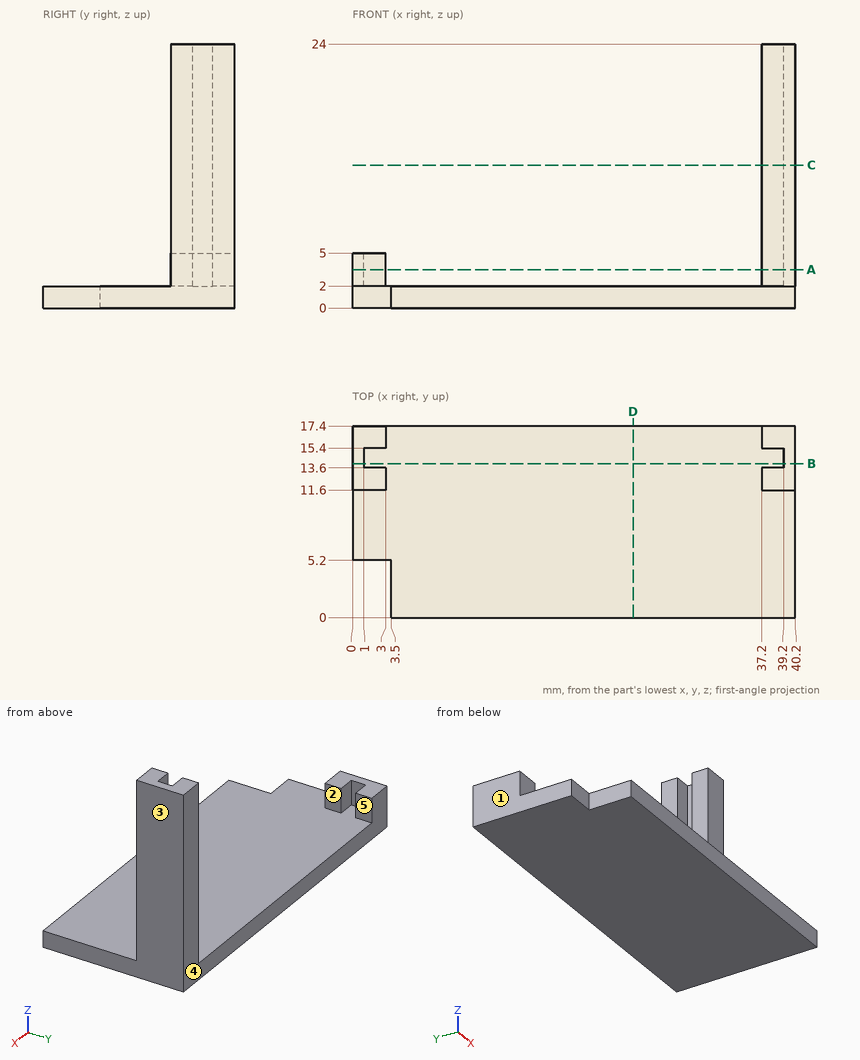
Check sheet for the drawn part. Datum: minimum x, y, z corner. Units: mm. A direction names the side the tool comes from. Give positions to 0.01 mm unless a question says otherwise; leave off trailing zeros. Order: outer loops, then holes, each group sorted by start corner. A loop starts at its lowest first (then second) coordinate and runs counter-clockwise, first axis right, second up. Notation, with made-up numbers: (-33, -12.75) -> (9, -12.75) arc R25 cw to (9, 14.25) -> close; hole circle Ø10 at (27, 66). An arc over 180 degrees is marked (long way). Return JSON: item names as keys, results as strings.
1. Go/stop test with flat-tipped pins: P1, Ø3.5, axis at x = 1, y = 13.5, coming from the +Z side; P2, Ø0.5, axis at y = 14.5, z = 9, coming from the -X side; P3, Ø0.6, axis at y = 17, z = 10.5, coming from the -X side; P4, Ø4, axis at x = 18, y = 15, coming from the -Z side. Record where each tip stops, or that it passes through.
From the geometry:
{"P1": "z = 5", "P2": "x = 39.2", "P3": "x = 37.2", "P4": "z = 0"}
2. Cross-section at A-A, the plane z = 3.5. Record the cut outline in (x, y).
From the geometry:
{"outline": "(0, 11.6) -> (3, 11.6) -> (3, 13.6) -> (1, 13.6) -> (1, 15.4) -> (3, 15.4) -> (3, 17.4) -> (0, 17.4) -> close; (37.2, 11.6) -> (40.2, 11.6) -> (40.2, 17.4) -> (37.2, 17.4) -> (37.2, 15.4) -> (39.2, 15.4) -> (39.2, 13.6) -> (37.2, 13.6) -> close"}
3. Cross-section at D-D, the plane x = 25.5. Record the cut outline in (y, z).
From the geometry:
{"outline": "(0, 0) -> (17.4, 0) -> (17.4, 2) -> (0, 2) -> close"}
4. Cross-section at C-C, the plane z = 13. Record the cut outline in (x, y), plus the area to 3 significant figures.
From the geometry:
{"outline": "(37.2, 11.6) -> (40.2, 11.6) -> (40.2, 17.4) -> (37.2, 17.4) -> (37.2, 15.4) -> (39.2, 15.4) -> (39.2, 13.6) -> (37.2, 13.6) -> close", "area": "13.8 mm^2"}
5. Set-up check for the marked faces 1 and 2: record each of +Z, -Z, +X, -X, +Y, -Y from which the full face is reachable in a straight line by a thin tool's end or side.
From the geometry:
{"face 1": "+Z, -Z, -X, +Y, -Y", "face 2": "+Z, +Y, -Y"}
6. Material ranges on probe 1 along X at (y, z) = (15.75, 3); probe 2 along Z at (x, y) = (8, 10.75); probe 3 along X at (y, z) = (14.5, 10.75), recorded low to high. Write a range as [from, to].
From the geometry:
{"probe 1": "[0, 3], [37.2, 40.2]", "probe 2": "[0, 2]", "probe 3": "[39.2, 40.2]"}
7. Cross-section at B-B, the plane y = 14. Record the cut outline in (x, z).
From the geometry:
{"outline": "(0, 0) -> (40.2, 0) -> (40.2, 24) -> (39.2, 24) -> (39.2, 2) -> (1, 2) -> (1, 5) -> (0, 5) -> close"}
8. Mould release check, pull along X, two halves, no side actions. Record for the marked faces 3, 4 and 5: +X half, -X half, draft (parallel to the pull), parting line (faces both ways), or undercut.
From the geometry:
{"face 3": "+X half", "face 4": "draft", "face 5": "undercut"}
